```python
from build123d import *

# Parameters (mm, degrees)
BOSS_EXTRUDE1_DEPTH = 3
SKETCH2_R           = 1.55
CUT_EXTRUDE1_DEPTH  = 356.879522089
BOSS_EXTRUDE3_START = -6
SKETCH3_R           = 1.55
BOSS_EXTRUDE3_DEPTH = 6
CHAMFER1_SIZE       = 1.6


with BuildPart() as part:
    # Sketch1 → Boss-Extrude1 (new body)
    with BuildSketch(Plane(origin=(0, 0, 0), x_dir=(1, 0, 0), z_dir=(0, 1, 0))):
        Polygon((5.02071, 249.35), (4.05, 248.379), (4.05, 235), (4.04962, 234.998), (4.04981, 234.996), (4.04812, 234.989), (4.04698, 234.983), (4.04588, 234.981), (4.04531, 234.979), (4.04157, 234.974), (4.0383, 234.968), (4.03662, 234.966), (4.03536, 234.965), (0.096072974, 231.02453611), (0.100466918, 230.999536627), (0.100466918, 10.040936627), (25.04559171, -14.896738024), (36.96279171, -14.896738024), (42.932604901, -8.925141349), (42.936204527, -8.922620814), (42.939004026, -8.919250398), (42.950303055, -8.91270872), (42.961001942, -8.905217131), (42.965301773, -8.904076493), (42.969093555, -8.901881205), (42.981993376, -8.899610189), (42.99459311, -8.896229197), (42.99899314, -8.896608851), (43.00329308, -8.895848512), (211.00329308, -8.895848512), (211.00729308, -8.896608512), (211.01229308, -8.896228512), (211.02429308, -8.899608512), (211.03729308, -8.901878512), (211.04129308, -8.904078512), (211.04529308, -8.905218512), (211.05629308, -8.912718512), (211.06729308, -8.919248512), (211.07029308, -8.922608512), (211.07446368, -8.9293432), (217.045710314, -14.898806454), (228.963710314, -14.898806454), (253.901184996, 10.046118309), (253.901184996, 230.963718309), (249.95959644, 234.904129665), (209.00059644, 234.904129665), (208.966596216, 234.910128396), (208.936595582, 234.927127275), (208.913594574, 234.954126417), (208.902593341, 234.987126006), (208.902593341, 235.021126006), (208.904592744, 235.029126155), (202.978707894, 240.953241173), (191.020707894, 240.953241173), (185.096592876, 235.027356323), (185.098592876, 235.019356323), (185.098592876, 234.985356323), (185.087592876, 234.952356323), (185.064592876, 234.925356323), (185.034592876, 234.908356323), (185.000592876, 234.902356323), (69.000592876, 234.902356323), (68.966392876, 234.908356323), (68.936292876, 234.925356323), (68.913992876, 234.952356323), (68.902092876, 234.985356323), (68.902092876, 235.019356323), (68.904890404, 235.027357188), (62.979005555, 240.951472206), (51.020405555, 240.951472206), (45.096290537, 235.025587356), (45.099090537, 235.017587356), (45.099090537, 234.983587356), (45.087190537, 234.950587356), (45.064890537, 234.923587356), (45.034790537, 234.906587356), (45.000590537, 234.900587356), (34.000590537, 234.900587356), (33.966390537, 234.906587356), (33.936290537, 234.923587356), (33.913990537, 234.950587356), (33.902090537, 234.983587356), (33.902090537, 235.017587356), (33.904888065, 235.025588221), (32.964897694, 235.965297853), (32.963697694, 235.966297853), (32.961997694, 235.968297853), (32.958697694, 235.974297853), (32.954997694, 235.979297853), (32.954400114, 235.981289787), (32.953300114, 235.983289787), (32.95219879, 235.989297006), (32.950499346, 235.996294719), (32.950699249, 235.998293754), (32.9503, 236.00029), (32.9503, 248.37929), (31.9793, 249.35), align=None)
    extrude(amount=BOSS_EXTRUDE1_DEPTH)

    # Sketch2 → Cut-Extrude1 (cut, through all)
    with BuildSketch(Plane(origin=(0, 3, 0), x_dir=(1, 0, 0), z_dir=(0, 1, 0))):
        with Locations(Location((17.00329308, 10.040936627, 0), (0, 0, 270))):
            Circle(SKETCH2_R)
        with Locations(Location((127.00329308, 10.040936627, 0), (0, 0, 270))):
            Circle(SKETCH2_R)
        with Locations(Location((232.003293088, 10.040936627, 0), (0, 0, 270))):
            Circle(SKETCH2_R)
        with Locations(Location((232.002032216, 115.040936627, 0), (0, 0, 270))):
            Circle(SKETCH2_R)
        with Locations(Location((232.000771344, 220.040936627, 0), (0, 0, 270))):
            Circle(SKETCH2_R)
        with Locations(Location((127.002032208, 115.040936627, 0), (0, 0, 270))):
            Circle(SKETCH2_R)
        with Locations(Location((17.00329308, 115.040936627, 0), (0, 0, 270))):
            Circle(SKETCH2_R)
        with Locations(Location((17.00329308, 220.040936627, 0), (0, 0, 270))):
            Circle(SKETCH2_R)
        with Locations(Location((127.000771337, 220.040936627, 0), (0, 0, 270))):
            Circle(SKETCH2_R)
        with Locations(Location((196.999707894, 231.003241173, 0), (0, 0, 270))):
            Circle(SKETCH2_R)
        with Locations(Location((56.999705555, 231.003241173, 0), (0, 0, 270))):
            Circle(SKETCH2_R)
        with Locations(Location((18.499978099, 242, 0), (0, 0, 270))):
            Circle(SKETCH2_R)
    extrude(amount=-CUT_EXTRUDE1_DEPTH, mode=Mode.SUBTRACT)

    # Sketch3 → Boss-Extrude3 (add)
    with BuildSketch(Plane.XZ.offset(BOSS_EXTRUDE3_START)):
        with Locations(Location((56.999705555, -231.003241173, 0), (0, 0, 270))):
            Circle(SKETCH3_R)
        with Locations(Location((196.999707894, -231.003241173, 0), (0, 0, 270))):
            Circle(SKETCH3_R)
    extrude(amount=BOSS_EXTRUDE3_DEPTH)

    # Chamfer1
    chamfer1_edges = [part.edges().sort_by_distance(p)[0] for p in [
        (232.000771344, 3, -221.590936627),
        (232.002032216, 3, -116.590936627),
        (232.003293088, 3, -11.590936627),
        (127.002032208, 3, -116.590936627),
        (17.00329308, 3, -116.590936627),
        (127.000771337, 3, -221.590936627),
        (17.00329308, 3, -221.590936627),
        (127.00329308, 3, -11.590936627),
        (17.00329308, 3, -11.590936627),
    ]]
    chamfer(chamfer1_edges, length=CHAMFER1_SIZE)


solid = part.part
```
CAD build for the part. Positions are in the model's coordinates, mm. A direction names the side the tool comes from. Coordinates: 2 decimals unless noted, no trailing zeros. Order: outer loops, then holes, each group sorted by start corner. A loop starts at its lowest first (then second) coordinate and runs counter-clockwise, first axis right, second up. Notation, with made-up numbers: (6, 17) - (58, 17) arc R26 cw to (58, 33) - close; hole circle Ø7 at (25.5, -27.5). An arc over 180 degrees is marked (long way). Use a Markdown table: item, result. Add a question column.
(1) Saw through at A-A (x = 168.5). Give the cut face in (y, z).
(2) Saw through at C-C (z = -145). Give the cut face in (x, y).
(3) Drill centre lines: line 1 along X through (y, z) = (2.05, -242); line 2 along Z through (x, y) = (138, 2.65); line 3 along X through (y, z) = (2.9, -224). Where is each one in solid material? Low to high. Write a range as [from, to].
(4) Which spindle directions (+Z, -Z, +X, -X, +Y, -Y) get a long thin tool onto all of the face, cutting with end or side? Do faces 1 (the face through (125, 0, -119)), 2 (the face through (39.91, 1.48, 11.95)), 3 (the face through (65.98, 1.48, -237.95)). Say none if no direction does.
(5) Flat gauge pins, fed straight in: pin 1 (1 mm diameter, centred on x = 224.5, y = 5, fed in from -Z); pin 2 (0.9 mm diameter, centred on x = 37.5, y = 1, fed in from -Z); pin 3 (4 mm diameter, centred on x = 135.5, z = -66, fed in from +Y); pin 4 (0.9 mm diameter, centred on y = 1, z = -84, fed in from -X). Where does each tip first touch, or does it go through?
(6) Saw through at B-B (y = 4.2). Give the cut face in (x, z).
Solved:
| question | item | result |
|---|---|---|
| 1 | outline | (0, -234.9) - (3, -234.9) - (3, 8.9) - (0, 8.9) - close |
| 2 | outline | (0.1, 0) - (253.9, 0) - (253.9, 3) - (0.1, 3) - close |
| 3 | line 1 | x = [4.05, 16.95], [20.05, 32.95] |
| 3 | line 2 | z = [-234.9, 8.9] |
| 3 | line 3 | x = [0.1, 253.9] |
| 4 | face 1 | +Z, -Z, +X, -X, -Y |
| 4 | face 2 | +Z, +Y, -Y |
| 4 | face 3 | -Z, +Y, -Y |
| 5 | pin 1 | passes through |
| 5 | pin 2 | stops at z = -234.9 |
| 5 | pin 3 | stops at y = 3 |
| 5 | pin 4 | stops at x = 0.1 |
| 6 | outline | circle Ø3.1 at (57, -231); circle Ø3.1 at (197, -231) |
